Read the model definition and answer for the solid it produces. Units are mm, in the model's axes. A direction names the side the tool comes from. Coordinates: 2 decimals unless noted, no trailing zeros. Loops run counter-clockwise (first coordinate to the right, second up) from the corner with the lowest first, then second, coordinate; pieces in that order, holes last. Notation, with made-up numbers: (56, 40) - (105, 40) arc R27 ccw to (105, 70) - close; hole circle Ø10 at (-13.5, 7.25). An arc over 180 degrees is marked (long way). One line per item, written item: value. Start each with the question number.
from build123d import *

# Parameters (mm, degrees)
SKETCH1_W           = 81
SKETCH1_H           = 81
BOSS_EXTRUDE1_DEPTH = 53
SKETCH2_R           = 35
BOSS_EXTRUDE2_DEPTH = 106
SKETCH3_R           = 5
BOSS_EXTRUDE3_DEPTH = 105
SKETCH4_R           = 2.55
BOSS_EXTRUDE4_DEPTH = 7.7
FILLET1_R           = 4
FILLET2_R           = 3
CUT_EXTRUDE1_START  = -84.5
SKETCH5_W           = 18.690524158
SKETCH5_H           = 8.031084599
CUT_EXTRUDE1_DEPTH  = 30
CUT_EXTRUDE2_START  = -32.7
CUT_EXTRUDE2_DEPTH  = 7.2


with BuildPart() as part:
    # Sketch1 → Boss-Extrude1 (new body)
    with BuildSketch(Plane.XY):
        with Locations((0, 15.5)):
            Rectangle(SKETCH1_W, SKETCH1_H)
    extrude(amount=BOSS_EXTRUDE1_DEPTH)

    # Sketch2 → Boss-Extrude2 (add)
    with BuildSketch(Plane.XY.offset(53)):
        with Locations((0, 15.5)):
            Circle(SKETCH2_R)
    extrude(amount=BOSS_EXTRUDE2_DEPTH)

    # Sketch3 → Boss-Extrude3 (add)
    with BuildSketch(Plane.XY):
        Circle(SKETCH3_R)
    extrude(amount=-BOSS_EXTRUDE3_DEPTH)

    # Sketch4 → Boss-Extrude4 (add)
    with BuildSketch(Plane.XY):
        with BuildLine():
            Line((-48.75, -25), (48.75, -25))
            ThreePointArc((48.75, -25), (54.755216961, -20.98744231), (53.346194078, -13.903805922))
            Line((53.346194078, -13.903805922), (40.5, -1.057611845))
            Line((40.5, -1.057611845), (40.5, 56))
            Line((40.5, 56), (-3.718974359, 56))
            Line((-3.718974359, 56), (-3.718974359, 59.910374765))
            ThreePointArc((-3.718974359, 59.910374765), (-10.368974359, 66.560374765), (-17.018974359, 59.910374765))
            Line((-17.018974359, 59.910374765), (-17.018974359, 56))
            Line((-17.018974359, 56), (-40.5, 56))
            Line((-40.5, 56), (-40.5, -1.057611845))
            Line((-40.5, -1.057611845), (-53.346194078, -13.903805922))
            ThreePointArc((-53.346194078, -13.903805922), (-54.755216961, -20.98744231), (-48.75, -25))
        make_face()
        with Locations(Location((-48.75, -18.5, 0), (0, 0, 180))):
            Circle(SKETCH4_R, mode=Mode.SUBTRACT)
        with Locations(Location((48.75, -18.5, 0), (0, 0, 180))):
            Circle(SKETCH4_R, mode=Mode.SUBTRACT)
        with Locations(Location((-10.368974359, 59.910374765, 0), (0, 0, 180))):
            Circle(SKETCH4_R, mode=Mode.SUBTRACT)
    extrude(amount=BOSS_EXTRUDE4_DEPTH)

    # Fillet1
    # the kernel refuses this fillet: 4 mm, written as the material it adds along each edge
    with BuildSketch(Plane(origin=(-17.018974359, 56, 0), x_dir=(-1, 0, 0), z_dir=(0, 0, 1))) as fillet1_piece_1:
        with BuildLine():
            CenterArc((3.999622872, -4), FILLET1_R, 90, 89.517820814)
            Line((-0.000235484, -3.96633794), (-0.400221319, -3.962971734))
            ThreePointArc((-0.400221319, -3.962971734), (-0.4, -3.910374765), (-0.4, 0))
            Line((-0.4, 0), (0, 0.4))
            Line((0, 0.4), (3.999622872, 0.4))
            Line((3.999622872, 0.4), (3.999622872, 0))
        make_face()
    extrude(amount=7.7)
    with BuildSketch(Plane(origin=(-3.718974359, 56, 0), x_dir=(1, 0, 0), z_dir=(0, 0, 1))) as fillet1_piece_2:
        with BuildLine():
            CenterArc((3.999622872, 4), FILLET1_R, 180.482179186, 89.517820814)
            Line((-0.000235484, 3.96633794), (-0.400221319, 3.962971734))
            ThreePointArc((-0.400221319, 3.962971734), (-0.4, 3.910374765), (-0.4, 0))
            Line((-0.4, 0), (0, -0.4))
            Line((0, -0.4), (3.999622872, -0.4))
            Line((3.999622872, -0.4), (3.999622872, 0))
        make_face()
    extrude(amount=7.7)

    # Fillet2
    fillet2_edges = [part.edges().sort_by_distance(p)[0] for p in [
        (40.5, 15.5, 53),
        (-35, 15.5, 159),
        (0, 56, 53),
        (-40.5, 15.5, 53),
        (-40.5, 56, 26.5),
        (40.5, 56, 26.5),
        (40.5, -25, 30.35),
        (-40.5, -25, 30.35),
        (0, -25, 53),
    ]]
    fillet(fillet2_edges, radius=FILLET2_R)

    # Sketch5 → Cut-Extrude1 (cut)
    with BuildSketch(Plane.XY.offset(CUT_EXTRUDE1_START)):
        with Locations((0.303510312, 7.3155423)):
            Rectangle(SKETCH5_W, SKETCH5_H)
    extrude(amount=-CUT_EXTRUDE1_DEPTH, mode=Mode.SUBTRACT)

    # Sketch6 → Cut-Extrude2 (cut)
    with BuildSketch(Plane.XY.offset(CUT_EXTRUDE2_START)):
        Polygon((8.240833127, 7.650995437), (8.240833127, 4), (-4, 4), (-4, -6.044194101), (-7.393498293, -6.044194101), (-7.393498293, 7.650995437), align=None)
    extrude(amount=-CUT_EXTRUDE2_DEPTH, mode=Mode.SUBTRACT)


solid = part.part
1) Straight lines are drawn through the part: L1, parallel to Z at x = 26, y = 19; L2, parallel to Y at x = -1.5, z = 80; L3, parallel to Y at x = 48, z = 3. For each, find the intervals that lie inside material, in ascending order.
2) Section C-C, the plane z = 113 is taken. Determine the outline of the cut face in (x, y), and give its area (3 significant figures).
3) Flat-ended cylindrical pins translate along their axes: P1, Ø6, axis at x = -10.37, y = 59.91, coming from the -Z side; P2, Ø0.5, axis at x = 1, y = 4.5, coming from the -Z side; P3, Ø15, axis at x = -14.5, z = 30.5, coming from the +Y side. Find the tip coordinate at first contact, or state that the pin passes through.
4) Section B-B, the plane z = -11.5 is taken. Determine the outline of the cut face in (x, y), and give its area (3 significant figures).
5) For faces 1 (the flat face through (0, 3.3, -95)), 2 (the flat face through (-34, 5, 53)), 3 (the flat face through (0, 4, -36)), determine the directions among +Z, -Z, +X, -X, +Y, -Y from which every point of the face is accessible in a straight line to the end or side of a thin tool.
6) Determine the mould class of faces 4 (the flat face through (0, 16, 159)), 5 (the cylindrical face through (-1.08, -4.88, -51.76)), 6 (the cylindrical face through (51.3, -18.6, 3.8)), 7 (the cylindrical face through (-10.04, 57.38, 3.8)) for opening direction Y: released by +Y, released by -Y, zero draft, split by the parting line, or undercut.
7) Section A-A, the plane y = 15.5 is taken. Determine the outline of the cut face in (x, z).
Answer below:
1. L1: 0 to 159
1. L2: -19.47 to 50.47
1. L3: -25 to -20.94, -16.06 to -8.56
2. outline: circle Ø70 at (0, 15.5)
2. area: 3,850 mm2
3. P1: z = 0
3. P2: z = -84.5
3. P3: y = 56
4. outline: circle Ø10 at (0, 0)
4. area: 78.5 mm2
5. face 1: -Z, +X, -X, +Y
5. face 2: +Z
5. face 3: +X, -X, +Y
6. face 4: zero draft
6. face 5: split by the parting line
6. face 6: undercut
6. face 7: undercut
7. outline: (-40.5, 0) - (40.5, 0) - (40.5, 50) arc R3 ccw to (37.5, 53) - (35, 53) - (35, 156) arc R3 ccw to (32, 159) - (-32, 159) arc R3 ccw to (-35, 156) - (-35, 53) - (-37.5, 53) arc R3 ccw to (-40.5, 50) - close
